Source: CAD feature listing. Evaluate the final solid. Frame: model axes, mm. A direction names the side the tool comes from. Give positions to 0.01 mm unless a question says otherwise; leave off trailing zeros. Order: outer loops, then holes, each group sorted by start corner. A loop starts at its lowest first (then second) coordinate and runs counter-clockwise, first axis right, second up.
1) Section B-B, the plane x = 10.5. Return loops of the section in (y, z), plus the area to 3 significant figures.
2) Material intervals for line 1 (X direction, y = 1.25, z = 42.5); line 2 (Z direction, x = -2, y = -0.5); line 3 (Y direction, x = 18.5, z = 13.5), sorted ascending.
3) Draft query along Z for faces 5 (the face through (-3, 9, 0)), 6 (the face through (-3, 3.338, 43)), 7 (the face through (10, 2, 40)), 8 (the face through (-3, 3.338, 7)). Return one class per face: released by +Z, released by -Z, zero draft, split by the parting line, or undercut.
4) First-contact query: P1, Ø1.6, axis at x = 11, y = 2, coming from the +Z side; P2, Ø10, axis at x = 16, y = 2, coming from the -Z side; P3, Ø8, axis at x = 11, z = 44.5, coming from the +Y side; P4, Ø0.6, axis at x = -3, z = 8, coming from the -Y side. Flat tips, straight axial feed; report the tip coordinate or a pass-through.
5) Section C-C, the plane y = 16.75. Return loops of the section in (x, z).
6) Section D-D, the plane x = 20.5. Return loops of the section in (y, z).
7) Access query for faces 1 (the face through (11, 1.338, 25)), 2 (the face through (11, 3.338, 25)), 3 (the face through (17.645, 2.324, 29.101)), 4 (the face through (-2.484, -0.211, 41.546)). Directions: +Z, -Z, +X, -X, +Y, -Y. A direction counts if a zero-diameter tool reaches every point of the face in a straight line with its end or side. Return the directions, or none.
```python
from build123d import *

# Parameters (mm, degrees)
EXTRUDE_1_DEPTH     = 50
SKETCH_2_W          = 24
SKETCH_2_H          = 10
SKETCH_2_W_2        = 14
SKETCH_2_H_2        = 4.5
CUT_EXTRUDE_1_DEPTH = 50
FILLET_1_R          = 2
FILLET_2_R          = 2
FILLET_3_R          = 2
FILLET_4_R          = 2
FILLET_5_R          = 2
FILLET_6_R          = 2
FILLET_7_R          = 2
FILLET_8_R          = 2
FILLET_9_R          = 2
FILLET_10_R         = 2
FILLET_11_R         = 2
FILLET_12_R         = 2
FILLET_14_R         = 2
FILLET_15_R         = 2
SKETCH_3_R          = 1
CUT_EXTRUDE_2_DEPTH = 7


with BuildPart() as part:
    # 草图1 → 凸台-拉伸1 (new body)
    with BuildSketch(Plane.XY):
        Polygon((-4.784615385, 19.338461538), (-4.784615385, -3.661538462), (-0.784615385, -3.661538462), (-0.784615385, 1.338461538), (23.215384615, 1.338461538), (23.215384615, 3.338461538), (-0.784615385, 3.338461538), (-0.784615385, 19.338461538), align=None)
    extrude(amount=EXTRUDE_1_DEPTH)

    # 草图2 → 切除-拉伸1 (cut)
    with BuildSketch(Plane(origin=(0, 3.338461538, 0), x_dir=(1, 0, 0), z_dir=(0, 1, 0))):
        with Locations((11.215384615, -45)):
            Rectangle(SKETCH_2_W, SKETCH_2_H)
        with Locations((11.215384615, -30.75)):
            Rectangle(SKETCH_2_W_2, SKETCH_2_H_2)
        with Locations((11.215384615, -19.25)):
            Rectangle(SKETCH_2_W_2, SKETCH_2_H_2)
        with Locations((11.215384615, -5)):
            Rectangle(SKETCH_2_W, SKETCH_2_H)
    extrude(amount=-CUT_EXTRUDE_1_DEPTH, mode=Mode.SUBTRACT)

    # 圆角1
    fillet_1_edges = [part.edges().sort_by_distance(p)[0] for p in [
        (23.215384615, 2.338461538, 40),
    ]]
    fillet(fillet_1_edges, radius=FILLET_1_R)

    # 圆角2
    fillet_2_edges = [part.edges().sort_by_distance(p)[0] for p in [
        (23.215384615, 2.338461538, 10),
    ]]
    fillet(fillet_2_edges, radius=FILLET_2_R)

    # 圆角3
    fillet_3_edges = [part.edges().sort_by_distance(p)[0] for p in [
        (4.215384615, 2.338461538, 28.5),
    ]]
    fillet(fillet_3_edges, radius=FILLET_3_R)

    # 圆角4
    fillet_4_edges = [part.edges().sort_by_distance(p)[0] for p in [
        (4.215384615, 2.338461538, 33),
    ]]
    fillet(fillet_4_edges, radius=FILLET_4_R)

    # 圆角5
    fillet_5_edges = [part.edges().sort_by_distance(p)[0] for p in [
        (4.215384615, 2.338461538, 17),
    ]]
    fillet(fillet_5_edges, radius=FILLET_5_R)

    # 圆角6
    fillet_6_edges = [part.edges().sort_by_distance(p)[0] for p in [
        (4.215384615, 2.338461538, 21.5),
    ]]
    fillet(fillet_6_edges, radius=FILLET_6_R)

    # 圆角7
    fillet_7_edges = [part.edges().sort_by_distance(p)[0] for p in [
        (18.215384615, 2.338461538, 17),
    ]]
    fillet(fillet_7_edges, radius=FILLET_7_R)

    # 圆角8
    fillet_8_edges = [part.edges().sort_by_distance(p)[0] for p in [
        (18.215384615, 2.338461538, 33),
    ]]
    fillet(fillet_8_edges, radius=FILLET_8_R)

    # 圆角9
    fillet_9_edges = [part.edges().sort_by_distance(p)[0] for p in [
        (18.215384615, 2.338461538, 28.5),
    ]]
    fillet(fillet_9_edges, radius=FILLET_9_R)

    # 圆角10
    fillet_10_edges = [part.edges().sort_by_distance(p)[0] for p in [
        (18.215384615, 2.338461538, 21.5),
    ]]
    fillet(fillet_10_edges, radius=FILLET_10_R)

    # 圆角11
    fillet_11_edges = [part.edges().sort_by_distance(p)[0] for p in [
        (-0.784615385, 19.338461538, 25),
    ]]
    fillet(fillet_11_edges, radius=FILLET_11_R)

    # 圆角12
    fillet_12_edges = [part.edges().sort_by_distance(p)[0] for p in [
        (-4.784615385, 19.338461538, 25),
    ]]
    fillet(fillet_12_edges, radius=FILLET_12_R - 0.0001)  # a hair under: the kernel refuses the full size

    # 圆角14
    fillet_14_edges = [part.edges().sort_by_distance(p)[0] for p in [
        (-2.784615385, -3.661538462, 50),
    ]]
    fillet(fillet_14_edges, radius=FILLET_14_R)

    # 圆角15
    fillet_15_edges = [part.edges().sort_by_distance(p)[0] for p in [
        (-2.784615385, -3.661538462, 0),
    ]]
    fillet(fillet_15_edges, radius=FILLET_15_R)

    # 草图3 → 切除-拉伸2 (cut)
    with BuildSketch(Plane.XZ.offset(3.661538462)):
        with Locations(Location((-2.784615385, 42.5, 0), (0, 0, 270))):
            Circle(SKETCH_3_R)
        with Locations(Location((-2.784615385, 7.5, 0), (0, 0, 90))):
            Circle(SKETCH_3_R)
    extrude(amount=-CUT_EXTRUDE_2_DEPTH, mode=Mode.SUBTRACT)


solid = part.part
```
From the geometry:
1. outline: (1.34, 10) - (3.34, 10) - (3.34, 17) - (1.34, 17) - close; (1.34, 21.5) - (3.34, 21.5) - (3.34, 28.5) - (1.34, 28.5) - close; (1.34, 33) - (3.34, 33) - (3.34, 40) - (1.34, 40) - close
1. area: 42.0 mm2
2. line 1: x = -4.78 to -3.78, -1.78 to -0.78
2. line 2: z = 0 to 6.88, 8.12 to 41.88, 43.12 to 50
2. line 3: y = 1.34 to 3.34
3. face 5: released by -Z
3. face 6: undercut
3. face 7: released by +Z
3. face 8: undercut
4. P1: stops at z = 40
4. P2: stops at z = 10
4. P3: passes through
4. P4: stops at y = 3.34
5. outline: (-4.78, 0) - (-0.78, 0) - (-0.78, 50) - (-4.78, 50) - close
6. outline: (1.34, 10) - (3.34, 10) - (3.34, 40) - (1.34, 40) - close
7. face 1: +Z, -Z, +X, -Y
7. face 2: +Z, -Z, +X, +Y
7. face 3: +Y, -Y
7. face 4: -Y
